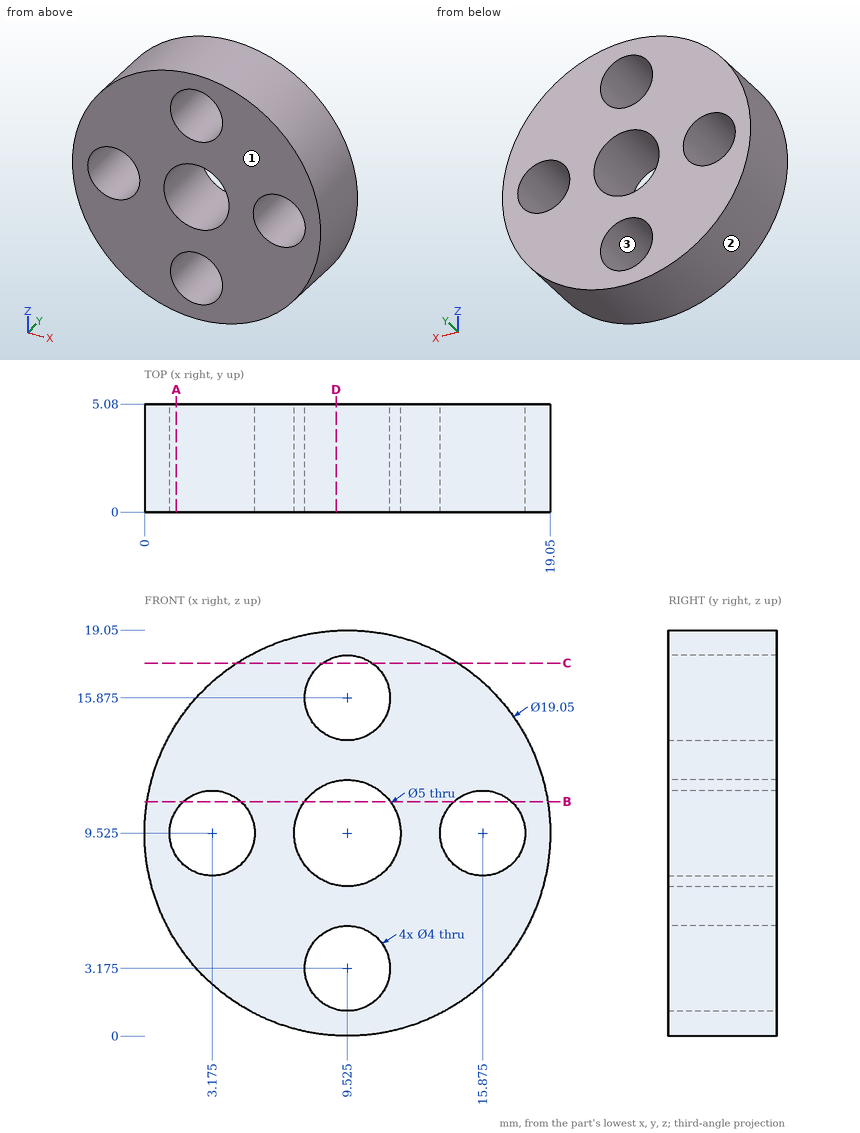
Here's the drawing with two shaded views (mm, measured from the low corner). I have some questions. Give positions to 0.01 mm unless a question says otherwise; leave off trailing zeros. Loops run counter-clockwise (first coordinate to the right, second up) from the corner with the lowest first, then second, coordinate; pieces in that order, holes last. Notation, with made-up numbers: M 21.5,18.5 L 70.5,18.5 A10 cw 70.5,34.5 Z; hole C -1.5,-13 d6. An arc over 180 degrees is marked long. Answer in a Markdown table with one row per item.
1. Suppose I cut it at C-C on z = 17.5. Write out the boundary of the cut face in (x, y).
Taken from the geometry:
| item | result |
|---|---|
| outline | M 4.32,0 L 8.36,0 L 8.36,5.08 L 4.32,5.08 Z; M 10.69,0 L 14.73,0 L 14.73,5.08 L 10.69,5.08 Z |
2. Thinking about a two-plate mould opening in Z: for the marked faces 1, 2 and 3, which applies, released by +Z, released by -Z, zero draft, split by the parting line, or undercut?
Taken from the geometry:
| item | result |
|---|---|
| face 1 | zero draft |
| face 2 | split by the parting line |
| face 3 | undercut |
3. If I drill on line 1 along Z through (x, y) = (9.25, 3.4); line 2 along X through (y, z) = (4.9, 8.5); line 3 along X through (y, z) = (0.45, 8), over which ranges is the centre line in solid material (lowest first)?
Taken from the geometry:
| item | result |
|---|---|
| line 1 | z = 0 to 1.19, 5.16 to 7.04, 12.01 to 13.89, 17.86 to 19.05 |
| line 2 | x = 0.06 to 1.46, 4.89 to 7.24, 11.81 to 14.16, 17.59 to 18.99 |
| line 3 | x = 0.12 to 1.88, 4.47 to 7.54, 11.51 to 14.58, 17.17 to 18.93 |
4. Suppose I cut it at D-D on x = 9. Write out the boundary of the cut face in (y, z).
Taken from the geometry:
| item | result |
|---|---|
| outline | M 0,0.01 L 5.08,0.01 L 5.08,1.25 L 0,1.25 Z; M 0,5.1 L 5.08,5.1 L 5.08,7.08 L 0,7.08 Z; M 0,11.97 L 5.08,11.97 L 5.08,13.95 L 0,13.95 Z; M 0,17.8 L 5.08,17.8 L 5.08,19.04 L 0,19.04 Z |
5. Suppose I cut it at B-B on z = 11. Write out the boundary of the cut face in (x, y), plus the area to 3 significant figures.
Taken from the geometry:
| item | result |
|---|---|
| outline | M 0.11,0 L 1.82,0 L 1.82,5.08 L 0.11,5.08 Z; M 4.53,0 L 7.51,0 L 7.51,5.08 L 4.53,5.08 Z; M 11.54,0 L 14.52,0 L 14.52,5.08 L 11.54,5.08 Z; M 17.23,0 L 18.94,0 L 18.94,5.08 L 17.23,5.08 Z |
| area | 47.7 mm² |
6. For pin 1 Ø1.5 at (y, z) = (4.5, 15.5) entering from +X; pin 2 Ø6.5 at (x, z) = (9.525, 15.875) entering from +Y; pin 3 Ø3 at (x, z) = (9.525, 3.175) entering from +Y, each with a flat end and sliding along its axis, tell me the tip position at first contact or that it passes through.
Taken from the geometry:
| item | result |
|---|---|
| pin 1 | stops at x = 17.49 |
| pin 2 | stops at y = 5.08 |
| pin 3 | passes through |
7. Suppose I cut it at A-A on x = 1.5. Write out the boundary of the cut face in (y, z).
Taken from the geometry:
| item | result |
|---|---|
| outline | M 0,4.39 L 5.08,4.39 L 5.08,8.43 L 0,8.43 Z; M 0,10.62 L 5.08,10.62 L 5.08,14.66 L 0,14.66 Z |
